Verification items for the finished model (mm, model axes). Coordinates: 2 decimals unless noted, no trailing zeros. Write each loop counter-clockwise with the first axis right and the second up, starting at its lowest first coordinate (ties: lowest second). Pieces come first, ordered by that corner, then holes. Notation, with made-up numbers: (34.5, 27) - (38.5, 27) arc R35 cw to (38.5, 63) - close; hole circle Ø8 at (-22.75, 22). An arc over 180 degrees is marked (long way). Use one line per item in the form item = value. Start each with the question number.
(1) Sectioned sample at D-D (z = -391). Record the cut outline in (x, y), and give its area (3 significant figures).
(2) Sectioned sample at C-C (y = 2.5). Record the cut outline in (x, z), and give its area (3 significant figures).
(3) Material ranges on line 1 (X direction, y = 1.65, z = -213.5); line 2 (X direction, y = 1.25, z = -174); line 3 (Z direction, x = -206, y = 0.3), recorded low to high. Write a range as [from, to].
(4) Gauge pin test, flat ends, axial feed: pin 1 Ø1 at (x, y) = (-11, 2) entering from -Z; pin 2 Ø1 at (x, y) = (-421, 1.5) entering from +Z; pin 3 Ø1.8 at (y, z) = (2, -411) entering from -X. Record the tip position at first contact, or that the pin passes through.
(5) Sectioned sample at A-A (z = -213.5). Record the cut outline in (x, y).
(6) Sectioned sample at B-B (x = -213.5). Record the cut outline in (y, z), and give its area (3 significant figures).
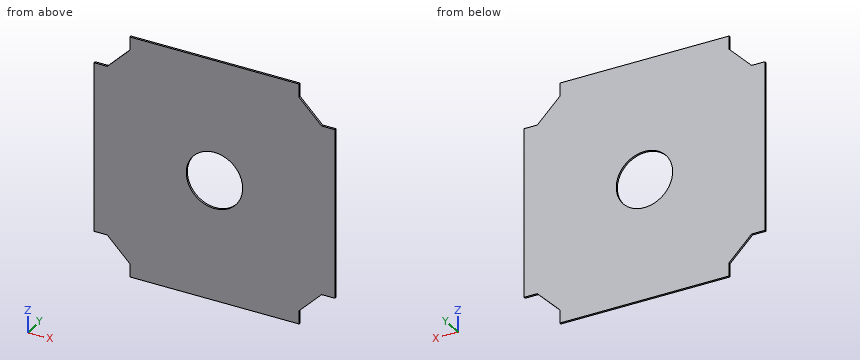
from build123d import *

# Parameters (mm, degrees)
BOSS_EXTRUDE1_DEPTH = 3.5
SKETCH2_R           = 50
CUT_EXTRUDE1_DEPTH  = 10


with BuildPart() as part:
    # Sketch1 → Boss-Extrude1 (new body)
    with BuildSketch(Plane(origin=(0, 0, 0), x_dir=(1, 0, 0), z_dir=(0, 1, 0))):
        Polygon((-363.5, 423.5), (-363.5, 403.5), (-403.5, 363.5), (-423.5, 363.5), (-427, 363.5), (-427, 63.5), (-423.5, 63.5), (-403.5, 63.5), (-363.5, 23.5), (-363.5, 3.5), (-363.5, 0), (-63.5, 0), (-63.5, 3.5), (-63.5, 23.5), (-23.5, 63.5), (-3.5, 63.5), (0, 63.5), (0, 363.5), (-3.5, 363.5), (-23.5, 363.5), (-63.5, 403.5), (-63.5, 423.5), (-63.5, 427), (-363.5, 427), align=None)
    extrude(amount=BOSS_EXTRUDE1_DEPTH)

    # Sketch2 → Cut-Extrude1 (cut)
    with BuildSketch(Plane(origin=(0, 3.5, 0), x_dir=(1, 0, 0), z_dir=(0, 1, 0))):
        with Locations(Location((-213.5, 213.5, 0), (0, 0, 270))):
            Circle(SKETCH2_R)
    extrude(amount=-CUT_EXTRUDE1_DEPTH, mode=Mode.SUBTRACT)


solid = part.part
Answers below:
q1.outline = (-376, 0) - (-51, 0) - (-51, 3.5) - (-376, 3.5) - close
q1.area = 1,140 mm2
q2.outline = (-427, -363.5) - (-403.5, -363.5) - (-363.5, -403.5) - (-363.5, -427) - (-63.5, -427) - (-63.5, -403.5) - (-23.5, -363.5) - (0, -363.5) - (0, -63.5) - (-23.5, -63.5) - (-63.5, -23.5) - (-63.5, 0) - (-363.5, 0) - (-363.5, -23.5) - (-403.5, -63.5) - (-427, -63.5) - close; hole circle Ø100 at (-213.5, -213.5)
q2.area = 162,000 mm2
q3.line_1 = [-427, -263.5], [-163.5, 0]
q3.line_2 = [-427, -244.16], [-182.84, 0]
q3.line_3 = [-427, -262.93], [-164.07, 0]
q4.pin_1 = -363.5
q4.pin_2 = -63.5
q4.pin_3 = -363.5
q5.outline = (-427, 0) - (-263.5, 0) - (-263.5, 3.5) - (-427, 3.5) - close; (-163.5, 0) - (0, 0) - (0, 3.5) - (-163.5, 3.5) - close
q6.outline = (0, -427) - (3.5, -427) - (3.5, -263.5) - (0, -263.5) - close; (0, -163.5) - (3.5, -163.5) - (3.5, 0) - (0, 0) - close
q6.area = 1,140 mm2
